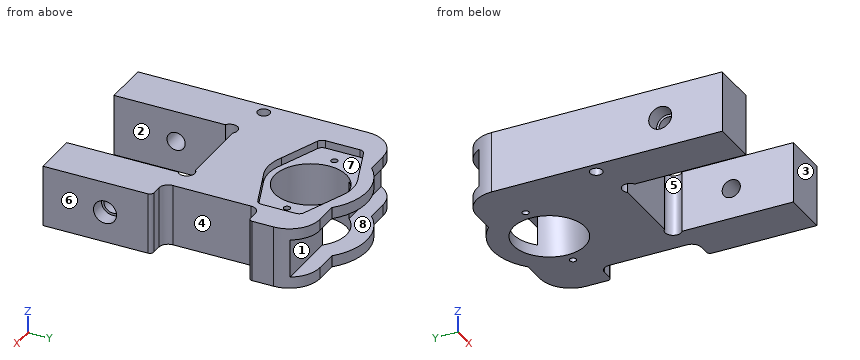
from build123d import *

# Parameters (mm, degrees)
SKETCH1_R               = 14.859
SKETCH1_R_2             = 2.5527
BOSS_EXTRUDE1_DEPTH     = 25.4
FILLET1_R               = 12.7
CUT_EXTRUDE1_DEPTH      = 3.175
FILLET2_R               = 2.54
SKETCH3_R               = 1.3462
CUT_EXTRUDE2_DEPTH      = 22.225
CUT_EXTRUDE3_START      = -76.2
SKETCH4_R               = 3.7703125
CUT_EXTRUDE3_DEPTH      = 76.2
SKETCH5_W               = 85.90580112
SKETCH5_H               = 15.875
CUT_EXTRUDE4_DEPTH      = 23.622
CUT_EXTRUDE4_DEPTH_BACK = 6.604
CUT_EXTRUDE5_START      = -25.4
SKETCH6_W               = 9.525
SKETCH6_H               = 39.923791379
CUT_EXTRUDE5_DEPTH      = 25.4
FILLET3_R               = 3.81
FILLET4_R               = 1.5875
SKETCH7_R               = 4.7625
CUT_EXTRUDE6_DEPTH      = 6.35


with BuildPart() as part:
    # Sketch1 → Boss-Extrude1 (new body)
    with BuildSketch(Plane.XY):
        with BuildLine():
            Line((38.1, -57.15), (19.05, -57.15))
            Line((19.05, -57.15), (19.05, -11.154684967))
            ThreePointArc((19.05, -11.154684967), (19.796266411, -6.337498405), (14.931562131, -6.026287555))
            Line((14.931562131, -6.026287555), (-14.931562131, -6.026287555))
            ThreePointArc((-14.931562131, -6.026287555), (-19.796266411, -6.337498405), (-19.05, -11.154684967))
            Line((-19.05, -11.154684967), (-19.05, -57.15))
            Line((-19.05, -57.15), (-38.1, -57.15))
            Line((-38.1, -57.15), (-38.1, 50.869712445))
            Line((-38.1, 50.869712445), (-15.983846846, 50.869712445))
            ThreePointArc((-15.983846846, 50.869712445), (0, 57.219712445), (15.983846846, 50.869712445))
            Line((15.983846846, 50.869712445), (38.1, 50.869712445))
            Line((38.1, 50.869712445), (38.1, -57.15))
        make_face()
        with Locations((0, 33.927912445)):
            Circle(SKETCH1_R, mode=Mode.SUBTRACT)
        with Locations((-33.3375, -2.611452402)):
            Circle(SKETCH1_R_2, mode=Mode.SUBTRACT)
        with Locations((33.3375, -2.611452402)):
            Circle(SKETCH1_R_2, mode=Mode.SUBTRACT)
    extrude(amount=BOSS_EXTRUDE1_DEPTH)

    # Fillet1
    fillet1_edges = [part.edges().sort_by_distance(p)[0] for p in [
        (-38.1, 50.869712445, 12.7),
        (38.1, 50.869712445, 12.7),
    ]]
    fillet(fillet1_edges, radius=FILLET1_R)

    # Sketch2 → Cut-Extrude1 (cut)
    with BuildSketch(Plane.XY.offset(25.4)):
        with BuildLine():
            Line((25.6921, 25.037912445), (25.6921, 42.817912445))
            Line((25.6921, 42.817912445), (7.274838916, 49.802912445))
            ThreePointArc((7.274838916, 49.802912445), (0, 51.390412445), (-7.274838916, 49.802912445))
            Line((-7.274838916, 49.802912445), (-25.6921, 42.817912445))
            Line((-25.6921, 42.817912445), (-25.6921, 25.037912445))
            Line((-25.6921, 25.037912445), (-7.274838916, 18.052912445))
            ThreePointArc((-7.274838916, 18.052912445), (0, 16.465412445), (7.274838916, 18.052912445))
            Line((7.274838916, 18.052912445), (25.6921, 25.037912445))
        make_face()
    extrude(amount=-CUT_EXTRUDE1_DEPTH, mode=Mode.SUBTRACT)

    # Fillet2
    fillet2_edges = [part.edges().sort_by_distance(p)[0] for p in [
        (-25.6921, 42.817912445, 23.8125),
        (25.6921, 42.817912445, 23.8125),
        (25.6921, 25.037912445, 23.8125),
        (-25.6921, 25.037912445, 23.8125),
    ]]
    fillet(fillet2_edges, radius=FILLET2_R)

    # Sketch3 → Cut-Extrude2 (cut)
    with BuildSketch(Plane.XY.offset(22.225)):
        with Locations((-19.05, 33.927912445)):
            Circle(SKETCH3_R)
        with Locations((19.05, 33.927912445)):
            Circle(SKETCH3_R)
    extrude(amount=-CUT_EXTRUDE2_DEPTH, mode=Mode.SUBTRACT)

    # Sketch4 → Cut-Extrude3 (cut)
    with BuildSketch(Plane.ZY.offset(38.1).offset(CUT_EXTRUDE3_START)):
        with Locations((12.7, -31.496)):
            Circle(SKETCH4_R)
    extrude(amount=CUT_EXTRUDE3_DEPTH, mode=Mode.SUBTRACT)

    # Sketch5 → Cut-Extrude4 (cut, two sides)
    with BuildSketch(Plane(origin=(0, 50.869712445, 0), x_dir=(1, 0, 0), z_dir=(0, 1, 0))) as cut_extrude4_sk:
        with Locations((0, -12.7)):
            Rectangle(SKETCH5_W, SKETCH5_H)
    extrude(amount=CUT_EXTRUDE4_DEPTH, mode=Mode.SUBTRACT)
    extrude(cut_extrude4_sk.sketch, amount=-CUT_EXTRUDE4_DEPTH_BACK, mode=Mode.SUBTRACT)

    # Sketch6 → Cut-Extrude5 (cut)
    with BuildSketch(Plane(origin=(0, 0, 0), x_dir=(-1, 0, 0), z_dir=(0, 0, -1)).offset(CUT_EXTRUDE5_START)):
        with Locations((-33.3375, 7.785139318)):
            Rectangle(SKETCH6_W, SKETCH6_H)
    extrude(amount=CUT_EXTRUDE5_DEPTH, mode=Mode.SUBTRACT)

    # Fillet3
    fillet3_edges = [part.edges().sort_by_distance(p)[0] for p in [
        (28.575, 27.747035008, 12.7),
        (28.575, -12.176756371, 12.7),
    ]]
    fillet(fillet3_edges, radius=FILLET3_R)

    # Fillet4
    fillet4_edges = [part.edges().sort_by_distance(p)[0] for p in [
        (38.1, -12.176756371, 12.7),
        (38.1, 27.747035008, 12.7),
    ]]
    fillet(fillet4_edges, radius=FILLET4_R)

    # Sketch7 → Cut-Extrude6 (cut)
    with BuildSketch(Plane(origin=(38.1, 0, 0), x_dir=(0, 0, -1), z_dir=(1, 0, 0))):
        with Locations((-12.7, -31.496)):
            Circle(SKETCH7_R)
    cut_extrude6 = extrude(amount=-CUT_EXTRUDE6_DEPTH, mode=Mode.SUBTRACT)

    # Mirror1: Cut-Extrude6 across plane
    add(cut_extrude6.mirror(Plane(origin=(0, 0, 0), x_dir=(0, 0, 1), z_dir=(1, 0, 0))), mode=Mode.SUBTRACT)


solid = part.part
CAD build for the part. Positions are in the model's coordinates, mm. Face numbers are marked on the shaded views. A direction names the side the tool comes from. Give positions to 0.01 mm unless a question says otherwise; leave off trailing zeros. Write each loop counter-clockwise with the first axis right and the second up, starting at its lowest first coordinate (ties: lowest second). Pieces come first, ordered by that corner, then holes. Notation, with made-up numbers: (25.5, 76) -> (42.5, 76) arc R6 ccw to (42.5, 80) -> close; hole circle Ø9 at (33, 4.25). An arc over 180 degrees is marked (long way). Return JSON: item names as keys, results as strings.
Item 1: Band-saw the part on A-A (x = 0). List the corners of the cut face in (y, z) (1 decimal), then the cut area to 3 significant figures.
Answer below:
{"outline": "(-6, 0) -> (19.1, 0) -> (19.1, 22.2) -> (16.5, 22.2) -> (16.5, 25.4) -> (-6, 25.4) -> close; (48.8, 0) -> (57.2, 0) -> (57.2, 4.8) -> (48.8, 4.8) -> close; (48.8, 20.6) -> (57.2, 20.6) -> (57.2, 25.4) -> (51.4, 25.4) -> (51.4, 22.2) -> (48.8, 22.2) -> close", "area": "701 mm2"}
Item 2: Band-saw the part on B-B (z = 19). Give the number of separate pieces and of enclosed holes in the cut face, then the cut area to 3 significant figures.
Answer below:
{"separate pieces": "1", "enclosed holes": "3", "area": "4,720 mm2"}
Item 3: Band-saw the part on C-C (x = -29.5). List the corners of the cut face in (y, z), then the cut area to 3 significant figures.
Answer below:
{"outline": "(-57.15, 0) -> (50.19, 0) -> (50.19, 4.76) -> (44.27, 4.76) -> (44.27, 20.64) -> (50.19, 20.64) -> (50.19, 25.4) -> (-57.15, 25.4) -> close; hole circle Ø7.54 at (-31.5, 12.7)", "area": "2,590 mm2"}
Item 4: Drill centre lines: probe 1 along Y at (x, z) = (34.25, 12.7); probe 2 along X at (y, z) = (-27, 10.5); probe 3 along Y at (x, z) = (34, 16.75). Where is each one in solid material? Low to high.
Answer below:
{"probe 1": "y = -57.15 to -36.26, -26.73 to -12.18, 27.75 to 44.27", "probe 2": "x = -38.1 to -19.05, 19.05 to 38.1", "probe 3": "y = -57.15 to -34, -28.99 to -12.18, 27.75 to 44.27"}
Item 5: Two-plate mould, pull along X, no slides. Class the marked faces 6, 7 and 8: +X half, -X half, draft (parallel to the pull), parting line (faces both ways), or undercut.
Answer below:
{"face 6": "+X half", "face 7": "undercut", "face 8": "draft"}
Item 6: Tool access for the marked faces 1, 2, 3, 4 and 5: list every direction of +Z, -Z, +X, -X, +Y, -Y with a clear straight run to the whole face (end or side of a thin tool).
Answer below:
{"face 1": "+X, -X, +Y", "face 2": "+Z, -Z, -Y", "face 3": "+Z, -Z, +X, -X, -Y", "face 4": "+Z, -Z, +X", "face 5": "+Z, -Z"}
Item 7: Drop flat-ended pins along their axis: pin 1 (2.5 mm diameter, centred on x = 20.5, z = 22, fed in from +Y); pin 2 (8.5 mm diameter, centred on y = -31.496, z = 12.7, fed in from -X); pin 3 (4.5 mm diameter, centred on y = -31.496, z = 12.7, fed in from -X); pin 4 (12 mm diameter, centred on x = -12.5, z = 3, fed in from -Y). Give the stop position or say it passes through.
Answer below:
{"pin 1": "stops at y = 50.87", "pin 2": "stops at x = -31.75", "pin 3": "passes through", "pin 4": "stops at y = -6.03"}
